The model under review builds one solid part; all positions refer to its coordinate system, in mm. Give positions to 0.01 mm unless a question says otherwise; leave off trailing zeros. Loops run counter-clockwise (first coordinate to the right, second up) from the corner with the lowest first, then second, coordinate; pieces in that order, holes last. Notation, with made-up numbers: M 88,-24.75 L 111,-24.75 A21 cw 111,2.25 Z; hole C -28,22.25 d1. An arc over 180 degrees is marked long. One line per item, written item: value. Start each with the question number.
Q1. We need section A-A on x = 36. Write out the cut boundary in (y, z), plus the area to 3 significant figures.
Q2. We need section C-C on z = 37.5. Write out the cut boundary in (x, y).
Q3. For pin 1 (6 mm diameter, centred on x = -6.5, y = -4, fed in from +Z); pin 2 (4 mm diameter, centred on x = 54.5, y = -10, fed in from +Z), all flat-tipped, find the tip position at first contact; note any pin that passes through.
Q4. To check wall thickness, follow line 1 along X through (y, z) = (-9.5, -43); line 2 along X through (y, z) = (-4.5, -49); line 3 along Z through (x, y) = (-46.5, -8.5). State the ranges of each line that lie inside material, in increasing order. Write a range as from..to.
Q5. We need section B-B on z = -60.5. Write out the cut boundary in (x, y).
Q6. We need section D-D on y = -8.5. Write out the cut boundary in (x, z), plus the area to 3 significant figures.
```python
from build123d import *

# Parameters (mm, degrees)
F1_DEPTH = 12.7


with BuildPart() as f1:
    # F0 (on Front) → F1 (new body)
    with BuildSketch(Plane.XZ):
        with BuildLine():
            ThreePointArc((6.572816, 6.812144), (26.277771, 47.8275), (61.812241, 76.250136))
            ThreePointArc((61.812241, 76.250136), (22.272642, 51.216691), (1.313443, 9.374544))
            ThreePointArc((1.313443, 9.374544), (-6.853136, 54.138947), (5.188448, 98.019979))
            ThreePointArc((5.188448, 98.019979), (-12.08547, 54.526704), (-4.447622, 8.356188))
            ThreePointArc((-4.447622, 8.356188), (-37.366378, 39.771156), (-53.417156, 82.349522))
            ThreePointArc((-53.417156, 82.349522), (-41.827343, 37.009369), (-8.509846, 4.146052))
            ThreePointArc((-8.509846, 4.146052), (-53.606934, 10.212135), (-91.619221, 35.224346))
            ThreePointArc((-91.619221, 35.224346), (-55.592593, 5.355713), (-9.321598, -1.647735))
            ThreePointArc((-9.321598, -1.647735), (-49.371463, -23.247574), (-94.825858, -25.355332))
            ThreePointArc((-94.825858, -25.355332), (-48.123361, -28.343643), (-6.572816, -6.812144))
            ThreePointArc((-6.572816, -6.812144), (-26.277771, -47.8275), (-61.812241, -76.250136))
            ThreePointArc((-61.812241, -76.250136), (-22.272642, -51.216691), (-1.313443, -9.374544))
            ThreePointArc((-1.313443, -9.374544), (6.853136, -54.138947), (-5.188448, -98.019979))
            ThreePointArc((-5.188448, -98.019979), (12.08547, -54.526704), (4.447622, -8.356188))
            ThreePointArc((4.447622, -8.356188), (37.366378, -39.771156), (53.417156, -82.349522))
            ThreePointArc((53.417156, -82.349522), (41.827343, -37.009369), (8.509846, -4.146052))
            ThreePointArc((8.509846, -4.146052), (53.606934, -10.212135), (91.619221, -35.224346))
            ThreePointArc((91.619221, -35.224346), (55.592593, -5.355713), (9.321598, 1.647735))
            ThreePointArc((9.321598, 1.647735), (49.371463, 23.247574), (94.825858, 25.355332))
            ThreePointArc((94.825858, 25.355332), (48.123361, 28.343643), (6.572816, 6.812144))
        make_face()
        Polygon((-4.938063, -1.002567), (-5.263817, 0), (-4.584271, 2.091427), (-4.258517, 3.093994), (-2.479443, 4.386567), (-1.626609, 5.006187), (0.572448, 5.006187), (1.626609, 5.006187), (3.405683, 3.713614), (4.258517, 3.093994), (4.938063, 1.002567), (5.263817, 0), (4.584271, -2.091427), (4.258517, -3.093994), (2.479443, -4.386567), (1.626609, -5.006187), (-0.572448, -5.006187), (-1.626609, -5.006187), (-3.405683, -3.713614), (-4.258517, -3.093994), align=None, mode=Mode.SUBTRACT)
        with BuildLine():
            ThreePointArc((-0.572448, -5.006187), (-0.250143, -2.507219), (0, 0))
            ThreePointArc((0, 0), (-1.676076, -1.881353), (-3.405683, -3.713614))
            Line((-3.405683, -3.713614), (-1.626609, -5.006187))
            Line((-1.626609, -5.006187), (-0.572448, -5.006187))
        make_face()
        with BuildLine():
            ThreePointArc((0, 0), (-2.461806, -0.536873), (-4.938063, -1.002567))
            Line((-4.938063, -1.002567), (-4.258517, -3.093994))
            Line((-4.258517, -3.093994), (-3.405683, -3.713614))
            ThreePointArc((-3.405683, -3.713614), (-1.676076, -1.881353), (0, 0))
        make_face()
        with BuildLine():
            Line((-4.584271, 2.091427), (-5.263817, 0))
            Line((-5.263817, 0), (-4.938063, -1.002567))
            ThreePointArc((-4.938063, -1.002567), (-2.461806, -0.536873), (0, 0))
            ThreePointArc((0, 0), (-2.307209, 1.012673), (-4.584271, 2.091427))
        make_face()
        with BuildLine():
            Line((-4.258517, 3.093994), (-4.584271, 2.091427))
            ThreePointArc((-4.584271, 2.091427), (-2.307209, 1.012673), (0, 0))
            ThreePointArc((0, 0), (-1.271337, 2.175413), (-2.479443, 4.386567))
            Line((-2.479443, 4.386567), (-4.258517, 3.093994))
        make_face()
        with BuildLine():
            ThreePointArc((-2.479443, 4.386567), (-1.271337, 2.175413), (0, 0))
            ThreePointArc((0, 0), (0.250143, 2.507219), (0.572448, 5.006187))
            Line((0.572448, 5.006187), (-1.626609, 5.006187))
            Line((-1.626609, 5.006187), (-2.479443, 4.386567))
        make_face()
        with BuildLine():
            ThreePointArc((0.572448, 5.006187), (0.250143, 2.507219), (0, 0))
            ThreePointArc((0, 0), (1.676076, 1.881353), (3.405683, 3.713614))
            Line((3.405683, 3.713614), (1.626609, 5.006187))
            Line((1.626609, 5.006187), (0.572448, 5.006187))
        make_face()
        with BuildLine():
            ThreePointArc((3.405683, 3.713614), (1.676076, 1.881353), (0, 0))
            ThreePointArc((0, 0), (2.461806, 0.536873), (4.938063, 1.002567))
            Line((4.938063, 1.002567), (4.258517, 3.093994))
            Line((4.258517, 3.093994), (3.405683, 3.713614))
        make_face()
        with BuildLine():
            ThreePointArc((4.938063, 1.002567), (2.461806, 0.536873), (0, 0))
            ThreePointArc((0, 0), (2.307209, -1.012673), (4.584271, -2.091427))
            Line((4.584271, -2.091427), (5.263817, 0))
            Line((5.263817, 0), (4.938063, 1.002567))
        make_face()
        with BuildLine():
            ThreePointArc((4.584271, -2.091427), (2.307209, -1.012673), (0, 0))
            ThreePointArc((0, 0), (1.271337, -2.175413), (2.479443, -4.386567))
            Line((2.479443, -4.386567), (4.258517, -3.093994))
            Line((4.258517, -3.093994), (4.584271, -2.091427))
        make_face()
        with BuildLine():
            ThreePointArc((2.479443, -4.386567), (1.271337, -2.175413), (0, 0))
            ThreePointArc((0, 0), (-0.250143, -2.507219), (-0.572448, -5.006187))
            Line((-0.572448, -5.006187), (1.626609, -5.006187))
            Line((1.626609, -5.006187), (2.479443, -4.386567))
        make_face()
    extrude(amount=F1_DEPTH)


solid = f1.part
```
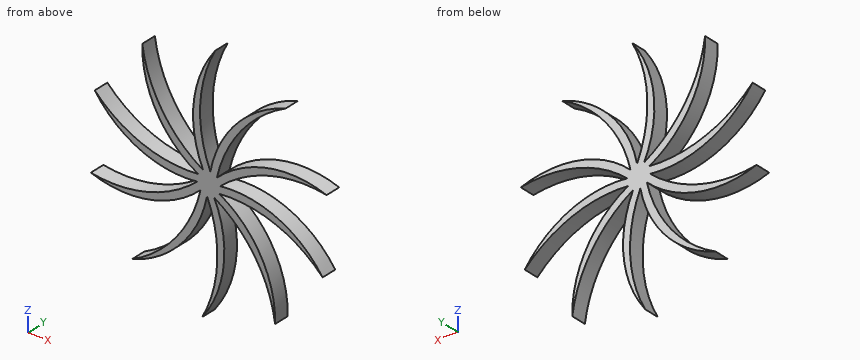
Solved:
1. outline: M -12.7,-37.76 L 0,-37.76 L 0,-28.15 L -12.7,-28.15 Z; M -12.7,-5.37 L 0,-5.37 L 0,0.78 L -12.7,0.78 Z; M -12.7,18.52 L 0,18.52 L 0,24.87 L -12.7,24.87 Z; M -12.7,58.43 L 0,58.43 L 0,63.5 L -12.7,63.5 Z
1. area: 345 mm2
2. outline: M -42.11,-12.7 L -35.82,-12.7 L -35.82,0 L -42.11,0 Z; M -12.25,-12.7 L -6.22,-12.7 L -6.22,0 L -12.25,0 Z; M 12.11,-12.7 L 19.05,-12.7 L 19.05,0 L 12.11,0 Z
3. pin 1: z = 83.99
3. pin 2: z = 74.46
4. line 1: -22.66..-15.69, 6.73..12.56, 39.42..44.97
4. line 2: -27.22..-20.33, 6.95..12.5, 42.8..47.55
4. line 3: -69.99..-67.12, -27.99..-22.41, 1.88..7.85, 46.41..56.91
5. outline: M -38.26,-12.7 L -32.08,-12.7 L -32.08,0 L -38.26,0 Z; M 6.38,-12.7 L 11.23,-12.7 L 11.23,0 L 6.38,0 Z; M 47.92,-12.7 L 51.11,-12.7 L 51.11,0 L 47.92,0 Z
6. outline: M -94.83,-25.36 A87.41 ccw -6.57,-6.81 A102.36 cw -61.81,-76.25 A87.41 ccw -1.31,-9.37 A102.36 cw -5.19,-98.02 A87.41 ccw 4.45,-8.36 A102.36 cw 53.42,-82.35 A87.41 ccw 8.51,-4.15 A102.36 cw 91.62,-35.22 A87.41 ccw 9.32,1.65 A102.36 cw 94.83,25.36 A87.41 ccw 6.57,6.81 A102.36 cw 61.81,76.25 A87.41 ccw 1.31,9.37 A102.36 cw 5.19,98.02 A87.41 ccw -4.45,8.36 A102.36 cw -53.42,82.35 A87.41 ccw -8.51,4.15 A102.36 cw -91.62,35.22 A87.41 ccw -9.32,-1.65 A102.36 cw Z
6. area: 4,400 mm2
